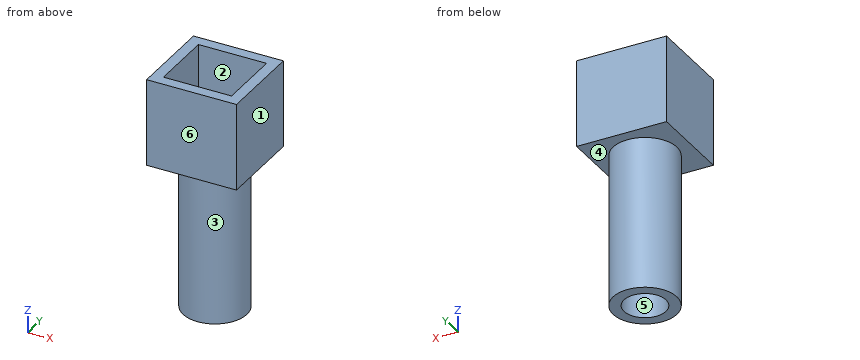
```python
from build123d import *

# Parameters (mm, degrees)
F0_R     = 2.925
F0_R_2   = 1.925
F1_DEPTH = 15
F3_W     = 8.25
F3_H     = 7.9
F3_W_2   = 6.25
F3_H_2   = 5.9
F3_R     = 2.925
F4_DEPTH = 1
F5_DEPTH = 7


with BuildPart() as f1:
    # F0 (on Top) → F1 (new body)
    with BuildSketch(Plane.XY):
        Circle(F0_R)
        Circle(F0_R_2, mode=Mode.SUBTRACT)
    extrude(amount=F1_DEPTH)

    # F3 (on face) → F4 (join)
    with BuildSketch(Plane.XY.offset(15)):
        Rectangle(F3_W, F3_H)
        Rectangle(F3_W_2, F3_H_2, mode=Mode.SUBTRACT)
        Rectangle(F3_W_2, F3_H_2)
        Circle(F3_R, mode=Mode.SUBTRACT)
    extrude(amount=-F4_DEPTH)

    # F3 (on face) → F5 (join)
    with BuildSketch(Plane.XY.offset(15)):
        Rectangle(F3_W, F3_H)
        Rectangle(F3_W_2, F3_H_2, mode=Mode.SUBTRACT)
    extrude(amount=F5_DEPTH)


solid = f1.part
```
CAD build for the part. Positions are in the model's coordinates, mm. Face numbers are marked on the shaded views. A direction names the side the tool comes from. Coordinates: 2 decimals unless noted, no trailing zeros. Write each loop counter-clockwise with the first axis right and the second up, starting at its lowest first coordinate (ties: lowest second). Pieces come first, ordered by that corner, then holes.
(1) Cut at D-D, the plane x = -2.5. List the corners of the cut face in (y, z).
(2) Drill centre lines: probe 1 along Y at (x, z) = (0, 11) (3 decimals); probe 2 along X at (y, z) = (2.25, 18.5) (3 decimals); probe 3 along Y at (x, z) = (-0.25, 21). Where is each one in solid material? Low to high.
(3) Cut at B-B, the plane x = 0. List the corners of the cut face in (y, z) (3 decimals).
(4) Cut at C-C, the plane z = 11.25. List the corners of the cut face in (x, y) (3 decimals), and give its area (3 significant figures).
(5) Two-plate mould, pull along Y, no slides. Class the marked faces 4, 5 and 6: +Y half, -Y half, draft (parallel to the pull), parting line (faces both ways), or undercut.
(6) Flat gauge pins, fed straight in: pin 1 (2 mm diameter, centred on y = 3, z = 3.5, fed in from +X); pin 2 (1 mm diameter, centred on x = 3, y = -3, fed in from -Z). Where does each tip first touch, or does it go through?
(7) Cut at A-A, the plane y = 0. List the corners of the cut face in (x, z) (3 decimals), and give its area (3 significant figures).
(8) 3-axis set-ups, long thin cutter, end or side, ignore diameter. For the marked faces 1, 2 and 3: which of +Z, -Z, +X, -X, +Y, -Y reach the whole face in a straight line?
Geometry says:
1. outline: (-3.95, 14) - (-1.52, 14) - (-1.52, 0) - (1.52, 0) - (1.52, 14) - (3.95, 14) - (3.95, 22) - (2.95, 22) - (2.95, 15) - (-2.95, 15) - (-2.95, 22) - (-3.95, 22) - close
2. probe 1: y = -2.925 to -1.925, 1.925 to 2.925
2. probe 2: x = -4.125 to -3.125, 3.125 to 4.125
2. probe 3: y = -3.95 to -2.95, 2.95 to 3.95
3. outline: (-3.95, 14) - (-2.925, 14) - (-2.925, 0) - (-1.925, 0) - (-1.925, 15) - (-2.95, 15) - (-2.95, 22) - (-3.95, 22) - close; (1.925, 0) - (2.925, 0) - (2.925, 14) - (3.95, 14) - (3.95, 22) - (2.95, 22) - (2.95, 15) - (1.925, 15) - close
4. outline: circle Ø5.85 at (0, 0); hole circle Ø3.85 at (0, 0)
4. area: 15.2 mm2
5. face 4: draft
5. face 5: undercut
5. face 6: -Y half
6. pin 1: stops at x = 2.13
6. pin 2: stops at z = 14
7. outline: (-4.125, 14) - (-2.925, 14) - (-2.925, 0) - (-1.925, 0) - (-1.925, 15) - (-3.125, 15) - (-3.125, 22) - (-4.125, 22) - close; (1.925, 0) - (2.925, 0) - (2.925, 14) - (4.125, 14) - (4.125, 22) - (3.125, 22) - (3.125, 15) - (1.925, 15) - close
7. area: 46.4 mm2
8. face 1: +Z, -Z, +X, +Y, -Y
8. face 2: +Z
8. face 3: -Z
